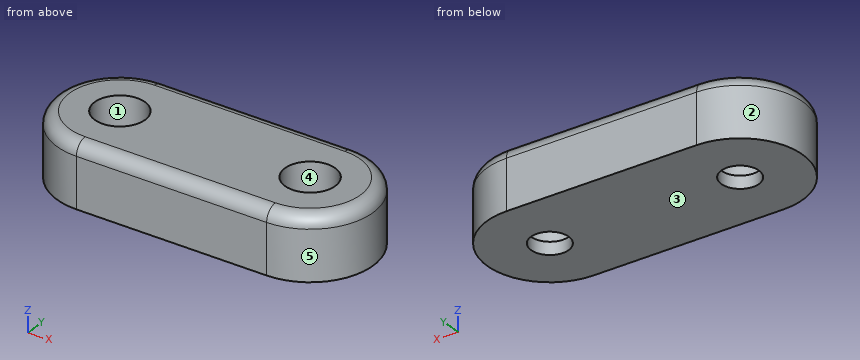
from build123d import *

# Parameters (mm, degrees)
SKETCH_R     = 1.5
PAD_DEPTH    = 5
SKETCH001_R  = 2
POCKET_DEPTH = 4
FILLET_R     = 1


with BuildPart() as part:
    # Sketch → Pad (new body)
    with BuildSketch(Plane.XY):
        with BuildLine():
            ThreePointArc((0, 5), (-5, 0), (0, -5))
            Line((0, -5), (15, -5))
            ThreePointArc((15, -5), (20, 0), (15, 5))
            Line((0, 5), (15, 5))
        make_face()
        Circle(SKETCH_R, mode=Mode.SUBTRACT)
        with Locations((15, 0)):
            Circle(SKETCH_R, mode=Mode.SUBTRACT)
    extrude(amount=PAD_DEPTH)

    # Sketch001 (on Face8 of Pad) → Pocket (cut)
    with BuildSketch(Plane.XY.offset(5)):
        Circle(SKETCH001_R)
        with Locations((15, 0)):
            Circle(SKETCH001_R)
    extrude(amount=-POCKET_DEPTH, mode=Mode.SUBTRACT)

    # Fillet
    fillet_edges = [part.edges().sort_by_distance(p)[0] for p in [
        (7.5, -5, 5),
    ]]
    fillet(fillet_edges, radius=FILLET_R)


solid = part.part
For this review, take the finished solid that the model builds, in its own axes (mm). Face numbers are marked on the shaded views. A direction names the side the tool comes from. Round coordinates to 2 decimals unless told otherwise and drop trailing zeros. Order: outer loops, then holes, each group sorted by start corner. A loop starts at its lowest first (then second) coordinate and runs counter-clockwise, first axis right, second up. Notation, with made-up numbers: M -5.5,3 L 42.5,3 A36 ccw 42.5,42 Z; hole C -2.75,-18 d9. An arc over 180 degrees is marked long. Write each question's results on one line, items separated by ' | '. Start each with the question number.
1. To check wall thickness, follow L1, parallel to X at y = 0, z = 0.35; L2, parallel to Y at x = 0, z = 3; L3, parallel to X at y = -1.75, z = 2.25. State the ranges of each line that lie inside material, in increasing order. Write a range as [from, to].
2. Add section A-A (y = 0). State the section outline as (x, z) points.
3. Draft analysis for pull direction Y (two halves, no side actions). For the marked faces 1, 2 and 3, state which applies: pulls with the +Y half, pulls with the -Y half, needs draft (parallel to the pull), parting line crosses it, or undercut.
4. Add section B-B (z = 2). State the section outline as (x, y) points.
5. Clearance check with flat-ended pins moving along their axes: pin 1 Ø1.5 at (y, z) = (-3.5, 3.5) entering from +X; pin 2 Ø1.2 at (x, y) = (16, -0.5) entering from +Z. State where each tip first meets the part, or that it passes through.
6. Tool access review of the marked faces 4 and 5: name each direction out of +Z, -Z, +X, -X, +Y, -Y from which nothing blocks a thin tool from reaching the whole face with its end or side.
Output values:
1) L1: [-5, -1.5], [1.5, 13.5], [16.5, 20] | L2: [-5, -2], [2, 5] | L3: [-4.68, -0.97], [0.97, 14.03], [15.97, 19.68]
2) outline: M -5,0 L -1.5,0 L -1.5,1 L -2,1 L -2,5 L -4,5 A1 ccw -5,4 Z; M 1.5,0 L 13.5,0 L 13.5,1 L 13,1 L 13,5 L 2,5 L 2,1 L 1.5,1 Z; M 16.5,0 L 20,0 L 20,4 A1 ccw 19,5 L 17,5 L 17,1 L 16.5,1 Z
3) face 1: undercut | face 2: parting line crosses it | face 3: needs draft
4) outline: M 0,-5 L 15,-5 A5 ccw 15,5 L 0,5 A5 ccw Z; hole C 0,0 d4; hole C 15,0 d4
5) pin 1: x = 19.18 | pin 2: z = 1
6) face 4: +Z | face 5: +Z, -Z, +X
